Source: CAD feature listing. Evaluate the final solid. Frame: model axes, mm. Round coordinates to 2 decimals unless told otherwise and drop trailing zeros. Loops run counter-clockwise (first coordinate to the right, second up) from the corner with the lowest first, then second, coordinate; pieces in that order, holes last. Notation, with made-up numbers: (15.5, 51.5) - (39.5, 51.5) arc R27 cw to (39.5, 69.5) - close; hole circle Ø8 at (10, -15). An arc over 180 degrees is marked (long way). Write item = value, one per line. Start each with the question number.
Autodesk Inventor part; units mm, degrees
ref_plane "YZ Plane" through (0, 0, 0) normal (1, 0, 0) x (0, 1, 0)
ref_plane "XZ Plane" through (0, 0, 0) normal (0, 1, 0) x (-1, 0, 0)
ref_plane "XY Plane" through (0, 0, 0) normal (0, 0, 1) x (1, 0, 0)
sketch "Sketch1" plane through (0, 0, 0) normal (0, 0, 1) x (1, 0, 0)
  circle A0 centre (0, 0) radius 5
  dimension "d0" = 10
extrude "Extrusion1" add sketch "Sketch1" along normal blind 50
sketch "Sketch2" plane through (0, 0, 50) normal (0, 0, 1) x (1, 0, 0)
  point P0 (0, 0)
  point P1 (0, 0)
sketch "Sketch3" plane through (0, 0, 0) normal (0, 0, -1) x (-1, 0, 0)
  point P0 (0, 0)
  point P1 (0, 0)
hole "Hole1" at (0, 0, 0) direction (0, 0, 1) diameter 2.459 depth 10 tip angle 118
hole "Hole2" at (0, 0, 50) direction (0, 0, -1) diameter 2.459 depth 10 tip angle 118
properties part number "SheetConnector"
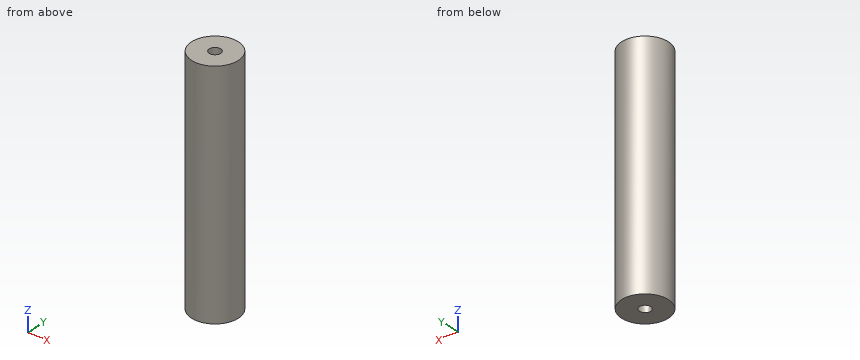
(1) Pin query (flat end, axial travel): P1, Ø1.5, axis at x = -2.5, z = 12.5, coming from the +Y side; P2, Ø2, axis at x = 0, y = 0, coming from the -Z side; P3, Ø1.5, axis at y = 3, z = 23, coming from the +X side. Return the tip coordinate at first contact, or that it passes through.
(2) Cut plane A-A (z = 43). Output: boundary loops of the cut face in (x, y).
(3) Material intervals for line 1 along Y through (x, z) = (0, 45); line 2 along Z through (x, y) = (1, -0.25); line 3 along X through (y, z) = (0.5, 9), sorted ascending. Write a range as from..to.
(4) Cut plane B-B (z = 25). Output: boundary loops of the cut face in (x, y), and give its area (3 significant figures).
(5) Cut plane C-C (y = 2). Output: boundary loops of the cut face in (x, z), and give its area (3 significant figures).
(6) Cut plane D-D (x = -4.5). Output: boundary loops of the cut face in (y, z).
Solution:
q1.P1 = 4.68
q1.P2 = 10.14
q1.P3 = 4.47
q2.outline = circle Ø10 at (0, 0); hole circle Ø2.46 at (0, 0)
q3.line_1 = -5..-1.23, 1.23..5
q3.line_2 = 10.12..39.88
q3.line_3 = -4.97..-1.12, 1.12..4.97
q4.outline = circle Ø10 at (0, 0)
q4.area = 78.5 mm^2
q5.outline = (-4.58, 0) - (4.58, 0) - (4.58, 50) - (-4.58, 50) - close
q5.area = 458 mm^2
q6.outline = (-2.18, 0) - (2.18, 0) - (2.18, 50) - (-2.18, 50) - close
